Answer from the drawing. Dimensions are ordinates in mm from the lowest x, y and z of the part. Give positions to 0.01 mm unless a question says otherwise; leave off trailing zeros. Write each loop counter-clockwise with the first axis right and the second up, starting at its lowest first coordinate (ties: lowest second). Pieces come first, ordered by that corner, then holes. Notation, with made-up numbers: (59.25, 39.5) - (77.25, 39.5) arc R17 ccw to (77.25, 68.5) - close; hole circle Ø7 at (58.5, -18.75). An arc over 180 degrees is marked (long way). Write item = value, one per line.
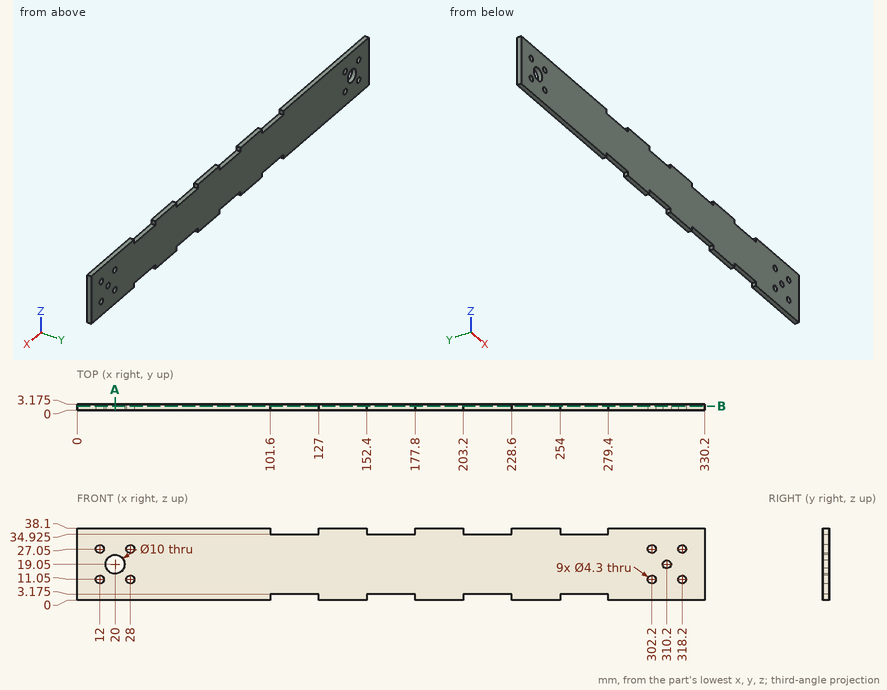
1. Find section B-B, the plane y = 2.1. Give the number of separate pieces and of enclosed holes in the cut face, then the cut area to 3 significant figures.
Solution:
separate_pieces = 1
enclosed_holes = 10
area = 11,700 mm^2
2. Given pin 1 (1.6 mm diameter, centred on x = 212.5, y = 2, fed in from -Z) (3 decimals); pin 2 (1 mm diameter, centred on x = 228, y = 2.5, fed in from +Z) (3 decimals), each flat-ended and moving along its own axis, determine where each tip first touches the part or whether it passes through.
Solution:
pin_1 = 3.175
pin_2 = 34.925
3. Straight lines are drawn through the part: line 1 (Z direction, x = 318.2, y = 2.4); line 2 (X direction, y = 1.5, z = 11.05); line 3 (X direction, y = 2.3, z = 19.05). For each, find the intervals that lie inside material, in ascending order.
Solution:
line_1 = 0 to 8.9, 13.2 to 24.9, 29.2 to 38.1
line_2 = 0 to 9.85, 14.15 to 25.85, 30.15 to 300.05, 304.35 to 316.05, 320.35 to 330.2
line_3 = 0 to 15, 25 to 308.05, 312.35 to 330.2
4. Find section A-A, the plane x = 20. Give the vertices of the cut face in (y, z) (3 decimals).
Solution:
outline = (0, 0) - (3.175, 0) - (3.175, 14.05) - (0, 14.05) - close; (0, 24.05) - (3.175, 24.05) - (3.175, 38.1) - (0, 38.1) - close
